Autodesk Inventor part; units mm, degrees
ref_plane "YZ Plane" through (0, 0, 0) normal (1, 0, 0) x (0, 1, 0)
ref_plane "XZ Plane" through (0, 0, 0) normal (0, 1, 0) x (-1, 0, 0)
ref_plane "XY Plane" through (0, 0, 0) normal (0, 0, 1) x (1, 0, 0)
sketch "Sketch2" plane through (0, 0, 0) normal (0, 0, 1) x (1, 0, 0)
  line L0 (0, 0) -> (-9.9, 0)
  line L1 (-9.9, 0) -> (-9.9, 105)
  line L2 (-9.9, 105) -> (0, 105)
  line L3 (0, 105) -> (0, 0)
  line L4 (-4.95, 0) -> (-4.95, 2.5)
  line L5 (-4.95, 0) -> (-2.45, 0) construction
  circle A0 centre (-4.95, 5) radius 2.5
  line L6 (-4.95, 7.5) -> (32.05, 7.5) construction
  line L7 (0, 44.5) -> (0, 0)
  line L8 (0, 0) -> (-9.9, 0)
  line L9 (-9.9, 0) -> (-9.9, 44.5)
  line L10 (0, 45.5) -> (0, 0)
  line L11 (0, 0) -> (-9.9, 0)
  line L12 (-9.9, 0) -> (-9.9, 45.5)
  line L13 (-4.95, 7.5) -> (66.05, 7.5) construction
  line L14 (-9.9, 78.5) -> (0, 78.5)
  dimension "d35" = 5
  dimension "d4" = 9.9
  dimension "d5" = 105
  dimension "d33" = 2.5
  dimension "d34" = 90
extrude "Extrusion5" add sketch "Sketch2" along normal blind 5 contours L0 L1 L14 L3
properties part number "Elbow_Cube_Holder_TestFit_V2"
Can you work these out from the model? Positions are in its coordinate system, mm. Coordinates: 2 decimals unless noted, no trailing zeros. Order: outer loops, then holes, each group sorted by start corner. A loop starts at its lowest first (then second) coordinate and runs counter-clockwise, first axis right, second up.
1. If we section it at B-B (y = 5): Please give me the cut outline in (x, z), then the cut area to 3 significant figures.
2. If we section it at A-A (x = -4.95): Please give me the cut outline in (y, z).
3. I'm going to push a flat-ended pin straight in: pin 1 (3 mm diameter, centred on x = -9, y = 54, fed in from -Z). Where does the tip first touch, or does it pass through?
4. If we section it at C-C (z = 0.8): Please give me the cut outline in (x, y), then the cut area to 3 significant figures.
5. I need wall thicknesses on line 1 (Y direction, x = -4.95, z = 1.6); line 2 (Y direction, x = -4.25, z = 4.5); line 3 (X direction, y = 5.5, z = 1.2). Which ranges of each line are inside material? Lowest first, please.
6. Thinking about a two-plate mould opening in Y: for faces 1 (the face through (0, 40, 2)), 2 (the face through (-5, 0, 2)), 3 (the face through (-2.565, 4.249, 2.465)), 4 (the face through (-5, 78.5, 2)), which applies, +Y half, -Y half, draft (parallel to the pull), parting line (faces both ways), or undercut?
Entries:
1. outline: (-9.9, 0) - (-7.45, 0) - (-7.45, 5) - (-9.9, 5) - close; (-2.45, 0) - (0, 0) - (0, 5) - (-2.45, 5) - close
1. area: 24.5 mm2
2. outline: (0, 0) - (2.5, 0) - (2.5, 5) - (0, 5) - close; (7.5, 0) - (78.5, 0) - (78.5, 5) - (7.5, 5) - close
3. pin 1: stops at z = 0
4. outline: (-9.9, 0) - (0, 0) - (0, 78.5) - (-9.9, 78.5) - close; hole circle Ø5 at (-4.95, 5)
4. area: 758 mm2
5. line 1: y = 0 to 2.5, 7.5 to 78.5
5. line 2: y = 0 to 2.6, 7.4 to 78.5
5. line 3: x = -9.9 to -7.4, -2.5 to 0
6. face 1: draft
6. face 2: -Y half
6. face 3: undercut
6. face 4: +Y half
